The drawing under review shows one solid part. Ordinate dimensions are in mm from its lowest x, y, z. Give positions to 0.01 mm unless a question says otherwise; leave off trailing zeros. Loops run counter-clockwise (first coordinate to the right, second up) from the corner with the lowest first, then second, coordinate; pieces in that order, holes last.
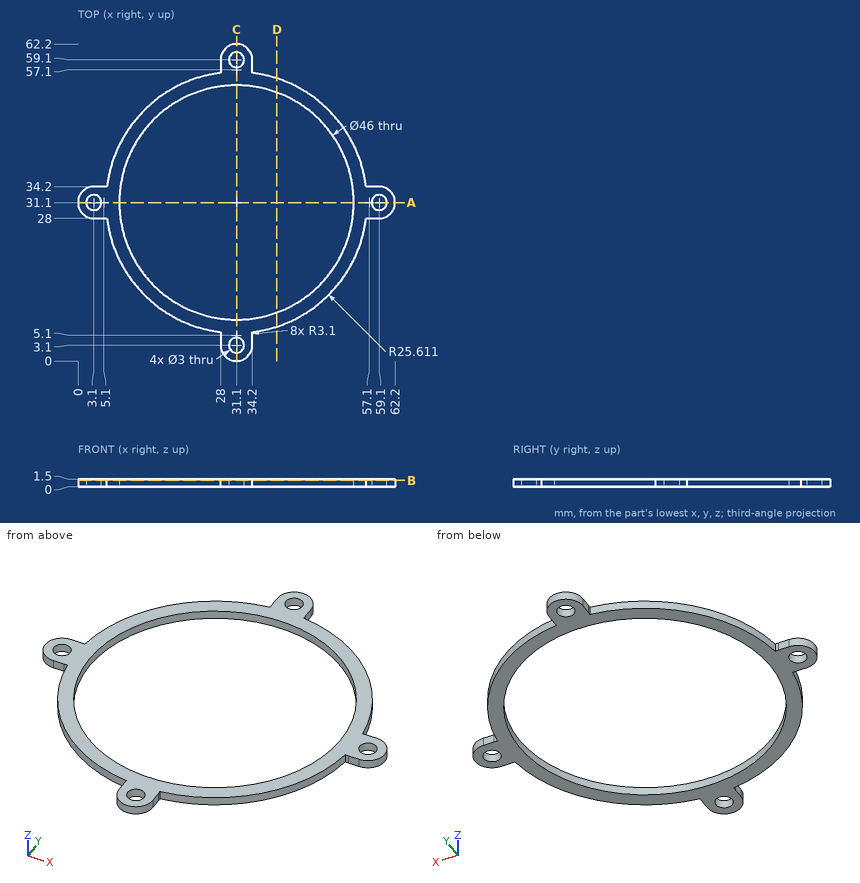
Item 1: Take a section at A-A on y = 31.1. Give the boundary of the cut face in (x, z).
Answer:
outline: (0, 0) - (1.6, 0) - (1.6, 1.5) - (0, 1.5) - close; (4.6, 0) - (8.1, 0) - (8.1, 1.5) - (4.6, 1.5) - close; (54.1, 0) - (57.6, 0) - (57.6, 1.5) - (54.1, 1.5) - close; (60.6, 0) - (62.2, 0) - (62.2, 1.5) - (60.6, 1.5) - close
Item 2: Take a section at B-B on z = 1.25. State how many separate pieces and enclosed holes the cut face has, and give its area (3 significant figures).
Answer:
separate pieces: 1
enclosed holes: 5
area: 492 mm2
Item 3: Clearance check with a flat-ended pin moving along its axis: pin 1 Ø2.5 at (x, y) = (31.1, 3.1) entering from +Z. State where the tip first meets the part, or that it passes through.
Answer:
pin 1: passes through
Item 4: Take a section at D-D on x = 39. Give the boundary of the cut face in (y, z).
Answer:
outline: (6.74, 0) - (9.5, 0) - (9.5, 1.5) - (6.74, 1.5) - close; (52.7, 0) - (55.46, 0) - (55.46, 1.5) - (52.7, 1.5) - close
Item 5: For L1, parallel to Y at x = 31.1, z = 0.55; L2, parallel to Y at x = 59.1, z = 0.65; L3, parallel to X at y = 31.5, z = 0.55, list the stretches that pass through material, from the lowest coordinate up.
Answer:
L1: y = 0 to 1.6, 4.6 to 8.1, 54.1 to 57.6, 60.6 to 62.2
L2: y = 28 to 29.6, 32.6 to 34.2
L3: x = 0.03 to 1.65, 4.55 to 8.1, 54.1 to 57.65, 60.55 to 62.17
